Autodesk Inventor part; units mm, degrees
ref_plane "YZ Plane" through (0, 0, 0) normal (1, 0, 0) x (0, 1, 0)
ref_plane "XZ Plane" through (0, 0, 0) normal (0, 1, 0) x (-1, 0, 0)
ref_plane "XY Plane" through (0, 0, 0) normal (0, 0, 1) x (1, 0, 0)
sketch "Sketch1" plane through (0, 0, 0) normal (0, 0, 1) x (1, 0, 0)
  line L0 (0, 0) -> (41.275, 0)
  line L1 (41.275, 0) -> (41.275, 25.4)
  line L2 (41.275, 25.4) -> (0, 25.4)
  line L3 (0, 25.4) -> (0, 0)
  circle A0 centre (6.35, 12.7) radius 2.0701
  line L4 (31.75, 18.1993) -> (36.5125, 15.4496)
  line L5 (36.5125, 15.4496) -> (36.5125, 9.9504)
  line L6 (36.5125, 9.9504) -> (31.75, 7.2007)
  line L7 (31.75, 7.2007) -> (26.9875, 9.9504)
  line L8 (26.9875, 9.9504) -> (26.9875, 15.4496)
  line L9 (26.9875, 15.4496) -> (31.75, 18.1993)
  circle A1 centre (19.05, 12.7) radius 2.0701
  point P0 (31.75, 12.7)
  dimension "d0" = 41.275
  dimension "d1" = 25.4
  dimension "d2" = 4.1402
  dimension "d3" = 12.7
  dimension "d4" = 6.35
  dimension "d5" = 25.4
  dimension "d6" = 9.525
  dimension "d7" = 12.7
  dimension "d13" = 12.7
extrude "Extrusion1" add sketch "Sketch1" along normal blind 3.175
fillet "Fillet1" radius 3.175 4 edges at (41.275, 25.4, 1.5875) (41.275, 0, 1.5875) (0, 25.4, 1.5875) (0, 0, 1.5875)
properties part number "Hex Spacer" material "Aluminum 6061"
Could you check a few things on this model? Use its own coordinates, in mm. A direction names the side the tool comes from. Round coordinates to 2 decimals unless told otherwise and drop trailing zeros. Order: outer loops, then holes, each group sorted by start corner. A loop starts at its lowest first (then second) coordinate and runs counter-clockwise, first axis right, second up.
(1) Imagine slicing it at A-A (y = 12.7). Write out the boundary of the cut face in (x, z) (1 decimal).
Response values:
outline: (0, 0) - (4.3, 0) - (4.3, 3.2) - (0, 3.2) - close; (8.4, 0) - (17, 0) - (17, 3.2) - (8.4, 3.2) - close; (21.1, 0) - (27, 0) - (27, 3.2) - (21.1, 3.2) - close; (36.5, 0) - (41.3, 0) - (41.3, 3.2) - (36.5, 3.2) - close
(2) If we mould it in two halves opening along X, with no side actions, what happens to faces 1 (the cylindrical face through (17, 13, 2)), 2 (the flat face through (41.275, 13, 2)), 3 (the flat face through (20, 10, 0)), 4 (the flat face through (26.988, 13, 2))? For each: released by +X, released by -X, zero draft, split by the parting line, or undercut.
Response values:
face 1: undercut
face 2: released by +X
face 3: zero draft
face 4: undercut
(3) Imagine slicing it at B-B (x = 19.05). Write out the boundary of the cut face in (y, z) (3 decimals), plus the area to 3 significant figures.
Response values:
outline: (0, 0) - (10.63, 0) - (10.63, 3.175) - (0, 3.175) - close; (14.77, 0) - (25.4, 0) - (25.4, 3.175) - (14.77, 3.175) - close
area: 67.5 mm2
(4) I'm going to push a flat-ended pin straight in: pin 1 (10 mm diameter, centred on x = 16.5, y = 14.5, fed in from -Z). Where does the tip first touch, or does it pass through?
Response values:
pin 1: stops at z = 0
(5) Imagine slicing it at D-D (x = 6.5). Write out the boundary of the cut face in (y, z) (3 decimals).
Response values:
outline: (0, 0) - (10.635, 0) - (10.635, 3.175) - (0, 3.175) - close; (14.765, 0) - (25.4, 0) - (25.4, 3.175) - (14.765, 3.175) - close
(6) Please list where these lines run through material, in increasing order: line 1 along X through (y, z) = (12.5, 1.7) (1 decimal); line 2 along Y through (x, z) = (6.35, 1.1); line 3 along X through (y, z) = (15.25, 1.7) (1 decimal).
Response values:
line 1: x = 0 to 4.3, 8.4 to 17, 21.1 to 27, 36.5 to 41.3
line 2: y = 0 to 10.63, 14.77 to 25.4
line 3: x = 0 to 27, 36.5 to 41.3
(7) Which directions (+Z, -Z, +X, -X, +Y, -Y) give clear straight access to the entire face, cutting with the end or side of a thin tool? Please do faces 5 (the cylindrical face through (0.95, 24.49, 1.61)), 6 (the flat face through (29.34, 16.81, 1.57)).
Response values:
face 5: +Z, -Z, -X, +Y
face 6: +Z, -Z
(8) Imagine slicing it at C-C (z = 0.7). Count the separate pieces of the cut face and the enclosed holes in it, plus the area to 3 significant figures.
Response values:
separate pieces: 1
enclosed holes: 3
area: 934 mm2
